Print and shaded views of the part. All mm, measured from the part's lowest x, y and z. Coordinates: 2 decimals unless noted, no trailing zeros. Loops run counter-clockwise (first coordinate to the right, second up) from the corner with the lowest first, then second, coordinate; pieces in that order, holes last. Notation, with made-up numbers: (-36, 41) -> (-22, 41) arc R12 cw to (-22, 58) -> close; hole circle Ø4 at (24, 19). An arc over 180 degrees is marked (long way). One line per item, written item: value. Start each with the question number.
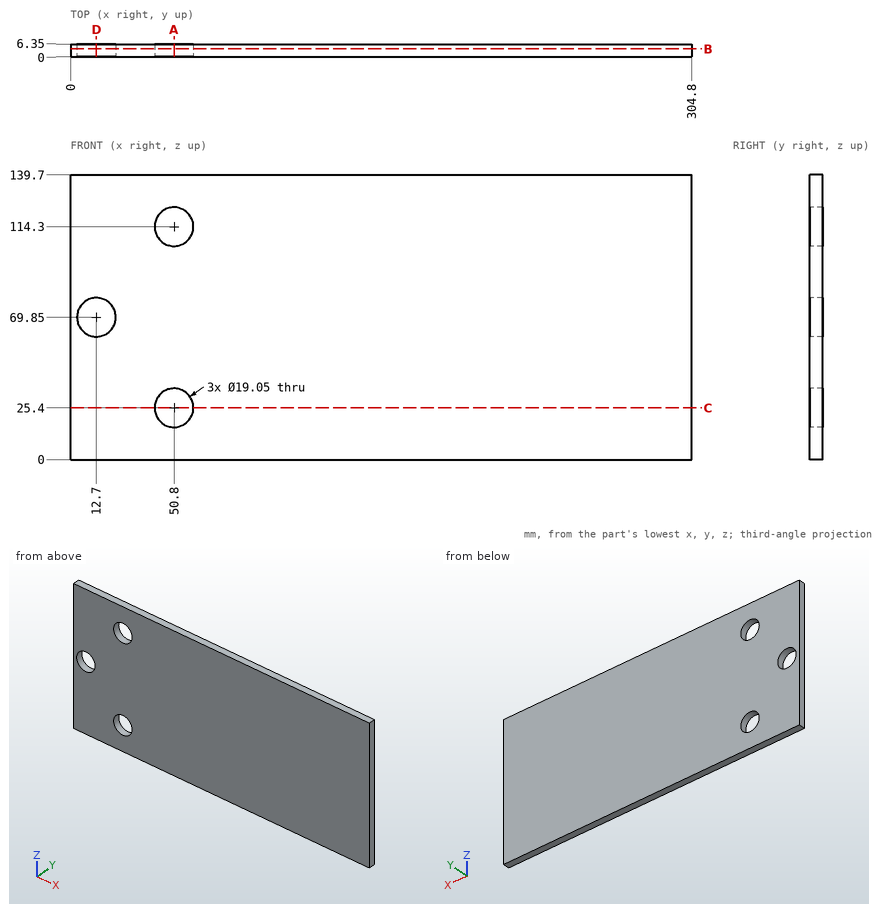
1) Slice it at B-B (y = 4). Give the cut face in (x, z) (3 decimals).
2) Slice it at C-C (z = 25.4). Give the cut face in (x, y) (3 decimals).
3) Slice it at A-A (x = 50.8). Give the cut face in (y, z) (3 decimals).
4) Slice it at D-D (x = 12.7). Give the cut face in (y, z) (3 decimals).
5) Pin check, flat tip, straight feed: pin 1 Ø1 at (x, y) = (47, 4.5) entering from -Z. Stop position of the tip, or through.
6) Probe line 1 (Z direction, x = 50.8, y = 2) (3 decimals); line 2 (X direction, y = 3.25, z = 114.3) (3 decimals); line 3 (Z direction, x = 12.7, y = 5) (3 decimals). List the from-to ranges inside material, lowest first. Write a range as from..to.
Check sheet entries:
1. outline: (0, 0) -> (304.8, 0) -> (304.8, 139.7) -> (0, 139.7) -> close; hole circle Ø19.05 at (12.7, 69.85); hole circle Ø19.05 at (50.8, 25.4); hole circle Ø19.05 at (50.8, 114.3)
2. outline: (0, 0) -> (41.275, 0) -> (41.275, 6.35) -> (0, 6.35) -> close; (60.325, 0) -> (304.8, 0) -> (304.8, 6.35) -> (60.325, 6.35) -> close
3. outline: (0, 0) -> (6.35, 0) -> (6.35, 15.875) -> (0, 15.875) -> close; (0, 34.925) -> (6.35, 34.925) -> (6.35, 104.775) -> (0, 104.775) -> close; (0, 123.825) -> (6.35, 123.825) -> (6.35, 139.7) -> (0, 139.7) -> close
4. outline: (0, 0) -> (6.35, 0) -> (6.35, 60.325) -> (0, 60.325) -> close; (0, 79.375) -> (6.35, 79.375) -> (6.35, 139.7) -> (0, 139.7) -> close
5. pin 1: stops at z = 0
6. line 1: z = 0..15.875, 34.925..104.775, 123.825..139.7
6. line 2: x = 0..41.275, 60.325..304.8
6. line 3: z = 0..60.325, 79.375..139.7
